Could you check a few things on this model? Use its own coordinates, in mm. A direction names the side the tool comes from. Give positions to 0.01 mm unless a question says otherwise; leave off trailing zeros. Order: outer loops, then holes, each group sorted by start corner. A loop starts at its lowest first (then second) coordinate and runs counter-clockwise, first axis right, second up.
(1) Imagine slicing it at C-C, the plane x = 64. Write out the boundary of the cut face in (y, z).
(2) On a 3-axis mill with a long thin cutter (end or side, diameter ignored), from which of +Z, -Z, +X, -X, +Y, -Y can I reach the whole of each face in a straight line? I mean faces 1 (the cylindrical face through (115.68, -0.783, 52.345)), 2 (the cylindrical face through (-102.85, -3.131, 71.493)), 3 (the cylindrical face through (-99.67, -4.78, -63.6)). Say none if no direction works.
(3) Imagine slicing it at B-B, the plane y = -5. State how many separate pieces and enclosed holes the cut face has, then the cut area to 3 significant figures.
(4) If I drill on probe 1 along X at (y, z) = (-0.25, -8); probe 2 along Z at (x, y) = (-73, -1.75); probe 3 along Z at (x, y) = (56.5, -0.75), over which ranges is the centre line in solid material (lowest first)?
(5) Imagine slicing it at A-A, the plane x = -36. Write out the boundary of the cut face in (y, z), then the cut area to 3 significant figures.
(6) If we mould it in two halves opening along Z, with no side actions, what happens to faces 4 (the cylindrical face through (128.281, -3.131, -70.935)), 5 (the cylindrical face through (-34.3, -3.13, -65.86)), 6 (the cylindrical face through (128.38, -3.131, 71.395)), 7 (the flat face through (-94, -3.175, -63))? For each: released by +Z, released by -Z, zero draft, split by the parting line, or undercut.
(7) Will these pins go through, and if not, where does the flat tip stop? pin 1 (12.5 mm diameter, centred on x = 12.72, z = 61.26, fed in from +Y); pin 2 (8.5 mm diameter, centred on x = 121.32, z = -60.7, fed in from -Y) (3 decimals).
from build123d import *

# Parameters (mm, degrees)
F0_R     = 2.38125
F0_R_2   = 4.7625
F1_DEPTH = 6.35
F2_R     = 4.7625
F3_DEPTH = 3.175
F5_DEPTH = 1.5875


with BuildPart() as f1:
    # F0 (on Front) → F1 (new body)
    with BuildSketch(Plane.XZ):
        with BuildLine():
            Line((123.840723, 73.304202), (-98.409277, 73.304202))
            ThreePointArc((-98.409277, 73.304202), (-102.899405, 71.44433), (-104.759277, 66.954202))
            Line((-104.759277, 66.954202), (-104.759277, -66.395798))
            ThreePointArc((-104.759277, -66.395798), (-102.899405, -70.885926), (-98.409277, -72.745798))
            Line((-98.409277, -72.745798), (123.840723, -72.745798))
            ThreePointArc((123.840723, -72.745798), (128.330851, -70.885926), (130.190723, -66.395798))
            Line((130.190723, -66.395798), (130.190723, 66.954202))
            ThreePointArc((130.190723, 66.954202), (128.330851, 71.44433), (123.840723, 73.304202))
        make_face()
        with Locations((-95.891841, -60.703362)):
            Circle(F0_R, mode=Mode.SUBTRACT)
        with Locations((-36.496777, -61.633298)):
            Circle(F0_R_2, mode=Mode.SUBTRACT)
        with Locations((12.719704, -60.703362)):
            Circle(F0_R, mode=Mode.SUBTRACT)
        with Locations((61.928223, -61.633298)):
            Circle(F0_R_2, mode=Mode.SUBTRACT)
        with Locations((121.323287, -60.703362)):
            Circle(F0_R, mode=Mode.SUBTRACT)
        with Locations((-98.409277, 0.279202)):
            Circle(F0_R, mode=Mode.SUBTRACT)
        with Locations((-95.891841, 61.261766)):
            Circle(F0_R_2, mode=Mode.SUBTRACT)
        with Locations((-72.757799, 61.261766)):
            Circle(F0_R, mode=Mode.SUBTRACT)
        with Locations((123.840723, 0.279202)):
            Circle(F0_R, mode=Mode.SUBTRACT)
        with Locations((12.719704, 61.261766)):
            Circle(F0_R, mode=Mode.SUBTRACT)
        with Locations((98.197206, 61.261766)):
            Circle(F0_R, mode=Mode.SUBTRACT)
        with Locations((121.323287, 61.261766)):
            Circle(F0_R_2, mode=Mode.SUBTRACT)
    extrude(amount=F1_DEPTH)

    # F2 (on face) → F3 (cut)
    with BuildSketch(Plane.XZ.offset(6.35)):
        with Locations((-98.409277, 0.279202)):
            Circle(F2_R)
        with Locations((12.719704, 61.261766)):
            Circle(F2_R)
        with Locations((123.840723, 0.279202)):
            Circle(F2_R)
        with Locations((121.323287, -60.703362)):
            Circle(F2_R)
        with Locations((12.719704, -60.703362)):
            Circle(F2_R)
        with Locations((-95.891841, -60.703362)):
            Circle(F2_R)
    extrude(amount=-F3_DEPTH, mode=Mode.SUBTRACT)

    # F4 (on face) → F5 (cut)
    with BuildSketch(Plane.XZ):
        with BuildLine():
            Line((117.490723, -47.345798), (117.490723, 47.904202))
            ThreePointArc((117.490723, 47.904202), (115.630851, 52.39433), (111.140723, 54.254202))
            Line((111.140723, 54.254202), (-85.709277, 54.254202))
            ThreePointArc((-85.709277, 54.254202), (-90.199405, 52.39433), (-92.059277, 47.904202))
            Line((-92.059277, 47.904202), (-92.059277, -47.345798))
            ThreePointArc((-92.059277, -47.345798), (-90.199405, -51.835926), (-85.709277, -53.695798))
            Line((-85.709277, -53.695798), (111.140723, -53.695798))
            ThreePointArc((111.140723, -53.695798), (115.630851, -51.835926), (117.490723, -47.345798))
        make_face()
        with BuildLine():
            ThreePointArc((111.140723, 51.079202), (113.385787, 50.149266), (114.315723, 47.904202))
            Line((114.315723, 47.904202), (114.315723, -47.345798))
            ThreePointArc((114.315723, -47.345798), (113.385787, -49.590862), (111.140723, -50.520798))
            Line((111.140723, -50.520798), (-85.709277, -50.520798))
            ThreePointArc((-85.709277, -50.520798), (-87.954341, -49.590862), (-88.884277, -47.345798))
            Line((-88.884277, -47.345798), (-88.884277, 47.904202))
            ThreePointArc((-88.884277, 47.904202), (-87.954341, 50.149266), (-85.709277, 51.079202))
            Line((-85.709277, 51.079202), (111.140723, 51.079202))
        make_face(mode=Mode.SUBTRACT)
    extrude(amount=F5_DEPTH, mode=Mode.SUBTRACT)


solid = f1.part
Answer block:
1. outline: (-6.35, -72.75) - (0, -72.75) - (0, -65.92) - (-6.35, -65.92) - close; (-6.35, -57.35) - (0, -57.35) - (0, -53.7) - (-1.59, -53.7) - (-1.59, -50.52) - (0, -50.52) - (0, 51.08) - (-1.59, 51.08) - (-1.59, 54.25) - (0, 54.25) - (0, 73.3) - (-6.35, 73.3) - close
2. face 1: +Y
2. face 2: +Z, -X, +Y, -Y
2. face 3: -Y
3. separate pieces: 1
3. enclosed holes: 12
3. area: 33,500 mm2
4. probe 1: x = -104.76 to -92.06, -88.88 to 114.32, 117.49 to 130.19
4. probe 2: z = -72.75 to 58.89, 63.63 to 73.3
4. probe 3: z = -72.75 to -53.7, -50.52 to 51.08, 54.25 to 73.3
5. outline: (-6.35, -72.75) - (0, -72.75) - (0, -66.37) - (-6.35, -66.37) - close; (-6.35, -56.9) - (0, -56.9) - (0, -53.7) - (-1.59, -53.7) - (-1.59, -50.52) - (0, -50.52) - (0, 51.08) - (-1.59, 51.08) - (-1.59, 54.25) - (0, 54.25) - (0, 73.3) - (-6.35, 73.3) - close
5. area: 857 mm2
6. face 4: released by -Z
6. face 5: undercut
6. face 6: released by +Z
6. face 7: undercut
7. pin 1: stops at y = 0
7. pin 2: stops at y = -3.175
